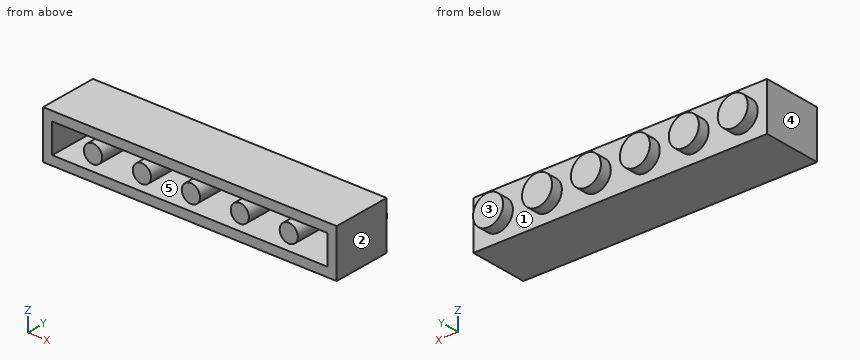
```python
from build123d import *

# Parameters (mm, degrees)
SKETCH1_W           = 47.85
SKETCH1_H           = 9.6
BOSS_EXTRUDE1_DEPTH = 7.78
SKETCH2_R           = 2.45
BOSS_EXTRUDE2_DEPTH = 1.89
SHELL1_T            = -1.5
SKETCH3_R           = 1.48
BOSS_EXTRUDE3_DEPTH = 7.9


with BuildPart() as part:
    # Sketch1 → Boss-Extrude1 (new body)
    with BuildSketch(Plane.XY):
        Rectangle(SKETCH1_W, SKETCH1_H)
    extrude(amount=-BOSS_EXTRUDE1_DEPTH)

    # Sketch2 → Boss-Extrude2 (add)
    with BuildSketch(Plane(origin=(0, 4.8, 0), x_dir=(1, 0, 0), z_dir=(0, 1, 0))):
        with Locations(Location((-19.9375, 3.89, 0), (0, 0, 90))):
            Circle(SKETCH2_R)
        with Locations(Location((-11.9625, 3.89, 0), (0, 0, 90))):
            Circle(SKETCH2_R)
        with Locations(Location((-3.9875, 3.89, 0), (0, 0, 90))):
            Circle(SKETCH2_R)
        with Locations(Location((3.9875, 3.89, 0), (0, 0, 90))):
            Circle(SKETCH2_R)
        with Locations(Location((11.9625, 3.89, 0), (0, 0, 90))):
            Circle(SKETCH2_R)
        with Locations(Location((19.9375, 3.89, 0), (0, 0, 90))):
            Circle(SKETCH2_R)
    extrude(amount=BOSS_EXTRUDE2_DEPTH)

    # Shell1
    shell1_openings = [part.faces().sort_by_distance(p)[0] for p in [
        (0, -4.8, -3.89),
    ]]
    offset(amount=SHELL1_T, openings=shell1_openings, kind=Kind.INTERSECTION)

    # Sketch3 → Boss-Extrude3 (add)
    with BuildSketch(Plane.XZ.offset(-3.3)):
        with Locations(Location((-15.95, -3.89, 0), (0, 0, 90))):
            Circle(SKETCH3_R)
        with Locations(Location((-7.975, -3.89, 0), (0, 0, 90))):
            Circle(SKETCH3_R)
        with Locations(Location((0, -3.89, 0), (0, 0, 90))):
            Circle(SKETCH3_R)
        with Locations(Location((7.975, -3.89, 0), (0, 0, 90))):
            Circle(SKETCH3_R)
        with Locations(Location((15.95, -3.89, 0), (0, 0, 90))):
            Circle(SKETCH3_R)
    extrude(amount=BOSS_EXTRUDE3_DEPTH)


solid = part.part
```
Here's how the part is built. I have some questions about the finished solid (model axes, mm). Face numbers are marked on the shaded views. A direction names the side the tool comes from. Give positions to 0.01 mm unless a question says otherwise; leave off trailing zeros. Order: outer loops, then holes, each group sorted by start corner. A loop starts at its lowest first (then second) coordinate and runs counter-clockwise, first axis right, second up. Notation, with made-up numbers: M 23.25,-6.5 L 68.25,-6.5 A28 ccw 68.25,15.5 Z; hole C -34.5,48.5 d2. An arc over 180 degrees is marked long. Use a Markdown table: item, result. Add a question column.
1. Suppose I cut it at A-A (y = -1). List the corners of the cut face in (x, z) for me (3 decimals), and give its area (3 significant figures).
2. I need wall thicknesses on probe 1 along Z at (x, y) = (-16, 2); probe 2 along Z at (x, y) = (-18.5, -1); probe 3 along Z at (x, y) = (-15, -1.75). Which ranges of each line are inside material? Lowest first, please. Write a range as from..to.
3. For pin 1 Ø0.9 at (x, z) = (7.5, -4) entering from -Y; pin 2 Ø1 at (x, y) = (-13, 5) entering from +Z; pin 3 Ø0.9 at (x, z) = (20.5, -3.5) entering from -Y; pin 4 Ø1 at (x, z) = (12, -3.5) entering from -Y, each with a flat end and sliding along its axis, tell me the tip position at first contact or that it passes through.
4. On a 3-axis mill with a long thin cutter (end or side, diameter ignored), from which of +Z, -Z, +X, -X, +Y, -Y can I reach the whole of each face in a straight line? I mean the marked faces 4 and 5. Say none if no direction works.
5. If we mould it in two halves opening along X, with no side actions, what happens to the marked faces 1, 2 and 3? For each: +X half, -X half, draft (parallel to the pull), parting line (faces both ways), or undercut.
6. Suppose I cut it at C-C (z = -0.75). List the corners of the cut face in (x, y) for me (3 decimals), and give its area (3 significant figures).
7. Suppose I cut it at B-B (x = 0). List the corners of the cut face in (y, z) for me.
8. Suppose I cut it at D-D (x = 17). List the corners of the cut face in (y, z) for me.
Results list:
| question | item | result |
|---|---|---|
| 1 | outline | M -23.925,-7.78 L 23.925,-7.78 L 23.925,0 L -23.925,0 Z; C -15.95,-3.89 d2.96; C -7.975,-3.89 d2.96; C 0,-3.89 d2.96; C 7.975,-3.89 d2.96; C 15.95,-3.89 d2.96; hole M -22.425,-6.28 L 22.425,-6.28 L 22.425,-1.5 L -22.425,-1.5 Z |
| 1 | area | 192 mm² |
| 2 | probe 1 | z = -7.78..-6.28, -5.37..-2.41, -1.5..0 |
| 2 | probe 2 | z = -7.78..-6.28, -1.5..0 |
| 2 | probe 3 | z = -7.78..-6.28, -5.02..-2.76, -1.5..0 |
| 3 | pin 1 | stops at y = -4.6 |
| 3 | pin 2 | stops at z = 0 |
| 3 | pin 3 | stops at y = 3.3 |
| 3 | pin 4 | stops at y = 5.19 |
| 4 | face 4 | +Z, -Z, -X, +Y, -Y |
| 4 | face 5 | -Y |
| 5 | face 1 | undercut |
| 5 | face 2 | +X half |
| 5 | face 3 | draft |
| 6 | outline | M -23.925,-4.8 L 23.925,-4.8 L 23.925,4.8 L -23.925,4.8 Z |
| 6 | area | 459 mm² |
| 7 | outline | M -4.8,-7.78 L 4.8,-7.78 L 4.8,0 L -4.8,0 L -4.8,-1.5 L 3.3,-1.5 L 3.3,-2.41 L -4.6,-2.41 L -4.6,-5.37 L 3.3,-5.37 L 3.3,-6.28 L -4.8,-6.28 Z |
| 8 | outline | M -4.8,-7.78 L 4.8,-7.78 L 4.8,0 L -4.8,0 L -4.8,-1.5 L 3.3,-1.5 L 3.3,-2.85 L -4.6,-2.85 L -4.6,-4.93 L 3.3,-4.93 L 3.3,-6.28 L -4.8,-6.28 Z |
